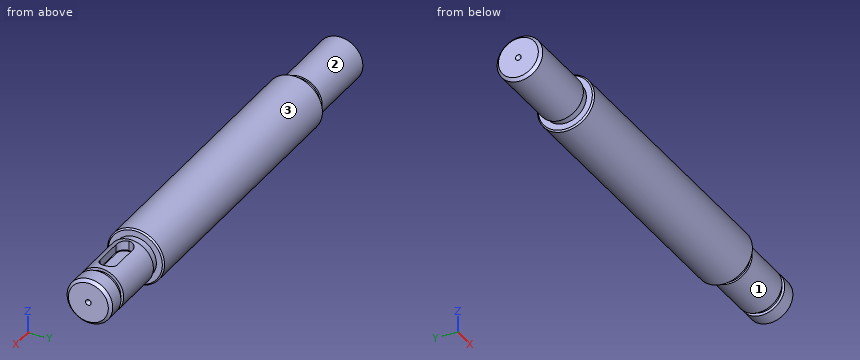
```python
from build123d import *

# Parameters (mm, degrees)
CHAMFER1_SIZE      = 0.5
SKETCH3_W          = 1.5
SKETCH3_H          = 0.3
SKETCH17_W         = 8
SKETCH17_H         = 3
CUT_EXTRUDE4_DEPTH = 1.8
FILLET10_R         = 1.5
FILLET11_R         = 1.5
FILLET12_R         = 0.1
SKETCH29_W         = 0.9
SKETCH29_H         = 0.5


with BuildPart() as part:
    # Sketch1 → Revolve1 (revolve)
    with BuildSketch(Plane.XY, mode=Mode.PRIVATE) as revolve1_sk:
        Polygon((0, 4), (15, 4), (15, 4.75), (15.25, 5), (65.75, 5), (66, 4.75), (66, 4), (81, 4), (81, 0), (0, 0), align=None)
    revolve(revolve1_sk.sketch.rotate(Axis((0, 0, 0), (1, 0, 0)), 90), axis=Axis((0, 0, 0), (1, 0, 0)))

    # Chamfer1
    chamfer1_edges = [part.edges().sort_by_distance(p)[0] for p in [
        (81, 0, -4),
        (0, 0, -4),
    ]]
    chamfer(chamfer1_edges, length=CHAMFER1_SIZE)

    # Sketch2 → Cut-Revolve1 (revolve, cut)
    with BuildSketch(Plane.XY, mode=Mode.PRIVATE) as cut_revolve1_sk:
        Polygon((0, 0.5), (0.5, 0), (0, 0), align=None)
        Polygon((81, 0), (81, 0.5), (80.5, 0), align=None)
    revolve(cut_revolve1_sk.sketch.rotate(Axis((0, 0, 0), (1, 0, 0)), 270), axis=Axis((0, 0, 0), (1, 0, 0)), mode=Mode.SUBTRACT)

    # Sketch3 → Cut-Revolve2 (revolve, cut)
    with BuildSketch(Plane.XY, mode=Mode.PRIVATE) as cut_revolve2_sk:
        with Locations((14.25, 3.85)):
            Rectangle(SKETCH3_W, SKETCH3_H)
        with Locations((66.75, 3.85)):
            Rectangle(SKETCH3_W, SKETCH3_H)
    revolve(cut_revolve2_sk.sketch.rotate(Axis((0, 0, 0), (1, 0, 0)), 90), axis=Axis((0, 0, 0), (1, 0, 0)), mode=Mode.SUBTRACT)

    # Sketch17 → Cut-Extrude4 (cut)
    with BuildSketch(Plane.XY.offset(4)):
        with Locations((72, 0)):
            Rectangle(SKETCH17_W, SKETCH17_H)
    extrude(amount=-CUT_EXTRUDE4_DEPTH, mode=Mode.SUBTRACT)

    # Fillet10
    fillet10_edges = [part.edges().sort_by_distance(p)[0] for p in [
        (76, 1.5, 2.954049622),
        (76, -1.5, 2.954049622),
    ]]
    fillet(fillet10_edges, radius=FILLET10_R - 0.0001)  # a hair under: the kernel refuses the full size

    # Fillet11
    fillet11_edges = [part.edges().sort_by_distance(p)[0] for p in [
        (68, 1.5, 2.954049622),
        (68, -1.5, 2.954049622),
    ]]
    fillet(fillet11_edges, radius=FILLET11_R - 0.0001)  # a hair under: the kernel refuses the full size

    # Fillet12
    fillet12_edges = [part.edges().sort_by_distance(p)[0] for p in [
        (72, 1.5, 2.2),
        (75.560689461, -1.060689461, 2.2),
        (75.560689461, 1.060689461, 2.2),
        (72, -1.5, 2.2),
        (68.439310539, -1.060689461, 2.2),
        (68.439310539, 1.060689461, 2.2),
    ]]
    fillet(fillet12_edges, radius=FILLET12_R)

    # Sketch29 → Cut-Revolve6 (revolve, cut)
    with BuildSketch(Plane.XY, mode=Mode.PRIVATE) as cut_revolve6_sk:
        with Locations((77.45, 3.75)):
            Rectangle(SKETCH29_W, SKETCH29_H)
    revolve(cut_revolve6_sk.sketch.rotate(Axis((81, 0, 0), (-1, 0, 0)), 270), axis=Axis((81, 0, 0), (-1, 0, 0)), mode=Mode.SUBTRACT)


solid = part.part
```
Here's how the part is built. I have some questions about the finished solid (model axes, mm). Face numbers are marked on the shaded views. A direction names the side the tool comes from. Coordinates: 2 decimals unless noted, no trailing zeros. Order: outer loops, then holes, each group sorted by start corner. A loop starts at its lowest first (then second) coordinate and runs counter-clockwise, first axis right, second up. Notation, with made-up numbers: (75, 7) - (110, 7) arc R19 cw to (110, 24) - close; hole circle Ø11 at (-39.75, 61). An arc over 180 degrees is marked (long way). One line per question, with ' | ' between items.
(1) For the marked faces 1, 2 and 3, which set-ups out of +Z, -Z, +X, -X, +Y, -Y let a thin tool reach every point of the face, with its end or its side?
Report:
face 1: +X | face 2: -X | face 3: +X, -X
(2) Suppose I cut it at A-A on x = 36. List the corners of the cut face in (y, z) for me, and give its area (3 significant figures).
Report:
outline: circle Ø10 at (0, 0) | area: 78.5 mm2
(3) Will these pins go through, and if not, where does the flat tip stop? pin 1 (1 mm diameter, centred on y = -3, z = 3, fed in from +X); pin 2 (1.5 mm diameter, centred on x = 71.5, z = 3, fed in from -Y); pin 3 (0.7 mm diameter, centred on x = 72.5, z = 3, fed in from +Y).
Report:
pin 1: stops at x = 80.76 | pin 2: stops at y = -3.31 | pin 3: stops at y = 3
(4) If I drill on L1, parallel to X at y = 2.5, z = 3; L2, parallel to X at y = 4.5, z = -1; L3, parallel to Y at x = 59, z = 3, over which ranges is the centre line in solid material (lowest first)?
Report:
L1: x = 0.41 to 13.5, 15 to 66, 67.5 to 77, 77.9 to 80.59 | L2: x = 15 to 66 | L3: y = -4 to 4
